Can you work these out from the model? Positions are in its coordinate system, mm. Give positions to 0.01 mm unless a question says otherwise; leave off trailing zeros. Order: outer loops, then holes, each group sorted by start corner. A loop starts at its lowest first (then second) coordinate and runs counter-clockwise, first axis right, second up. Notation, with made-up numbers: (53, -35) -> (111, -35) arc R36 cw to (111, 2) -> close; hole circle Ø1 at (88, -24). An arc over 180 degrees is marked (long way). Answer as a JSON object with one key per item and string values.
```python
from build123d import *

# Parameters (mm, degrees)
EXTRUSION1_DEPTH = 323
ESQUISSE2_R      = 1.5
EXTRUSION2_DEPTH = 248
ESQUISSE3_R      = 1.5
EXTRUSION3_DEPTH = 248


with BuildPart() as part:
    # Esquisse1 → Extrusion1 (new body)
    with BuildSketch(Plane.XY):
        Polygon((-20.61337059, 2.046), (-20.61337059, -12.954), (-5.61337059, -12.954), (-5.61337059, -11.454), (-19.11337059, -11.454), (-19.11337059, 2.046), align=None)
    extrude(amount=EXTRUSION1_DEPTH)

    # Esquisse2 → Extrusion2 (cut)
    with BuildSketch(Plane(origin=(0, -11.454, 0), x_dir=(-1, 0, 0), z_dir=(0, 1, 0))):
        with Locations((13.11337059, 7.5)):
            Circle(ESQUISSE2_R)
        with Locations((10.11337059, 274)):
            Circle(ESQUISSE2_R)
        with Locations((13.11337059, 315.5)):
            Circle(ESQUISSE2_R)
        with Locations((13.11337059, 231)):
            Circle(ESQUISSE2_R)
    extrude(amount=-EXTRUSION2_DEPTH, mode=Mode.SUBTRACT)

    # Esquisse3 → Extrusion3 (cut)
    with BuildSketch(Plane(origin=(-19.11337059, 0, 0), x_dir=(0, 0, -1), z_dir=(1, 0, 0))):
        with Locations((-36.5, -5.454)):
            Circle(ESQUISSE3_R)
        with Locations((-274, -3.954)):
            Circle(ESQUISSE3_R)
        with Locations((-315.5, -5.454)):
            Circle(ESQUISSE3_R)
    extrude(amount=-EXTRUSION3_DEPTH, mode=Mode.SUBTRACT)


solid = part.part
```
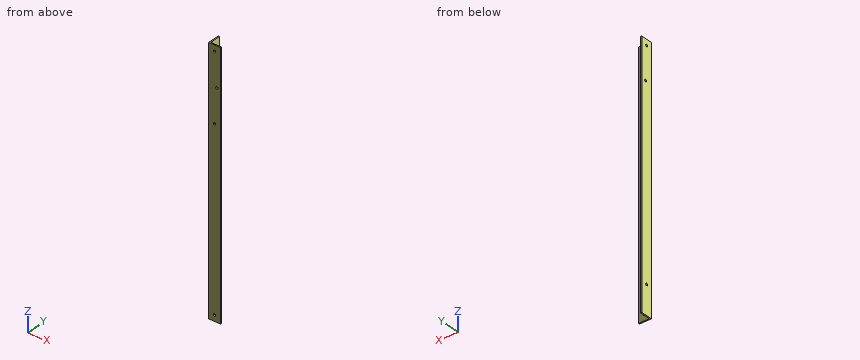
1. If we section it at A-A on z = 244.5: Please give me the cut outline in (x, y).
Worked answers:
{"outline": "(-20.61, -12.95) -> (-5.61, -12.95) -> (-5.61, -11.45) -> (-19.11, -11.45) -> (-19.11, 2.05) -> (-20.61, 2.05) -> close"}
2. Will these pins go through, and if not, where does the flat tip stop? pin 1 Ø4 at (x, z) = (-10.5, 162.5) entering from +Y; pin 2 Ø4 at (y, z) = (-5.5, 159.5) entering from +X.
Worked answers:
{"pin 1": "y = -11.45", "pin 2": "x = -19.11"}
3. Please list where these lines run through material, in increasing order: L1, parallel to X at y = -7.25, z = 221.5; L2, parallel to Y at x = -16.75, z = 120; L3, parallel to X at y = -12.55, z = 315.5.
Worked answers:
{"L1": "-20.61 to -19.11", "L2": "-12.95 to -11.45", "L3": "-20.61 to -14.61, -11.61 to -5.61"}
